```python
from build123d import *

# Parameters (mm, degrees)
SKETCH1_W           = 20
SKETCH1_H           = 6
BOSS_EXTRUDE1_DEPTH = 75
SKETCH2_W           = 20
SKETCH2_H           = 8
BOSS_EXTRUDE2_DEPTH = 26
SKETCH3_W           = 20
SKETCH3_H           = 6
BOSS_EXTRUDE3_DEPTH = 10
SKETCH6_W           = 13
SKETCH6_H           = 13
CUT_EXTRUDE1_DEPTH  = 79.014421744
SKETCH8_R           = 1.5
CUT_EXTRUDE3_DEPTH  = 5
CUT_EXTRUDE4_START  = -5
SKETCH9_R           = 1.5
CUT_EXTRUDE4_DEPTH  = 5
FILLET1_R           = 2
SKETCH10_W          = 6
SKETCH10_H          = 44.050587659
CUT_EXTRUDE5_DEPTH  = 20


with BuildPart() as part:
    # Sketch1 → Boss-Extrude1 (new body)
    with BuildSketch(Plane(origin=(0, 0, 0), x_dir=(1, 0, 0), z_dir=(0, 1, 0))):
        with Locations((-17.5, 0)):
            Rectangle(SKETCH1_W, SKETCH1_H)
    extrude(amount=BOSS_EXTRUDE1_DEPTH)

    # Sketch2 → Boss-Extrude2 (add)
    with BuildSketch(Plane.XY.offset(3)):
        with Locations((-17.5, 71)):
            Rectangle(SKETCH2_W, SKETCH2_H)
    extrude(amount=BOSS_EXTRUDE2_DEPTH)

    # Sketch3 → Boss-Extrude3 (add)
    with BuildSketch(Plane.XZ.offset(-67)):
        with Locations((-17.5, 26)):
            Rectangle(SKETCH3_W, SKETCH3_H)
    extrude(amount=BOSS_EXTRUDE3_DEPTH)

    # Sketch6 → Cut-Extrude1 (cut, through all)
    with BuildSketch(Plane.XZ.offset(-67)):
        with Locations((-17.5, 13)):
            Rectangle(SKETCH6_W, SKETCH6_H)
    extrude(amount=-CUT_EXTRUDE1_DEPTH, mode=Mode.SUBTRACT)

    # Sketch8 → Cut-Extrude3 (cut)
    with BuildSketch(Plane.XY.offset(6.5)):
        with Locations((-17.5, 71)):
            Circle(SKETCH8_R)
    extrude(amount=-CUT_EXTRUDE3_DEPTH, mode=Mode.SUBTRACT)

    # Sketch9 → Cut-Extrude4 (cut)
    with BuildSketch(Plane(origin=(0, 0, 19.5), x_dir=(-1, 0, 0), z_dir=(0, 0, -1)).offset(CUT_EXTRUDE4_START)):
        with Locations(Location((17.5, 71, 0), (0, 0, 180))):
            Circle(SKETCH9_R)
    extrude(amount=CUT_EXTRUDE4_DEPTH, mode=Mode.SUBTRACT)

    # Fillet1
    fillet1_edges = [part.edges().sort_by_distance(p)[0] for p in [
        (-17.5, 67, 3),
        (-17.5, 67, 23),
    ]]
    fillet(fillet1_edges, radius=FILLET1_R)

    # Sketch10 → Cut-Extrude5 (cut)
    with BuildSketch(Plane(origin=(-7.5, 0, 0), x_dir=(0, 0, -1), z_dir=(1, 0, 0))):
        with Locations((0, 21.22470617)):
            Rectangle(SKETCH10_W, SKETCH10_H)
    extrude(amount=-CUT_EXTRUDE5_DEPTH, mode=Mode.SUBTRACT)


solid = part.part
```
Input: part model. Units: mm. Frame: model coordinates. A direction names the side the tool comes from. Round coordinates to 2 decimals unless told otherwise and drop trailing zeros. Order: outer loops, then holes, each group sorted by start corner. A loop starts at its lowest first (then second) coordinate and runs counter-clockwise, first axis right, second up. Notation, with made-up numbers: (34, -9) - (91, -9) arc R29 cw to (91, 20) - close; hole circle Ø2 at (-27.75, 60.5). An arc over 180 degrees is marked (long way). One line per question, with ' | ' between items. Start each with the question number.
1) Cut plane A-A, the plane x = -14.25. Return the cut outline in (y, z).
2) Set-up query: faces 1 (the flat face through (-18, 57, 26)), 2 (the flat face through (-18, 61, 23)), 3 (the flat face through (-18, 71, 1.5)), 4 (the flat face through (-19, 72, 19.5)). Return all of +Z, -Z, +X, -X, +Y, -Y with unobstructed straight access to the full face (end or side cutting, diameter ignored); none if empty.
3) Cut plane C-C, the plane z = 15. Return the cut outline in (x, y).
4) Contact query for flat-ended pins moving along their axis: P1, Ø5, axis at x = -21, z = 27, coming from the -Y side; P2, Ø1, axis at x = -10, z = 10.5, coming from the -Y side. Output: stop coordinate, or through.
5) Cut plane D-D, the plane y = 71. Return the cut outline in (x, z).
6) Cut plane B-B, the plane y = 62.5. Return the cut outline in (x, z), then the cut area to 3 significant figures.
7) Pull-direction query (X, two-part tool) for faces 5 (the flat face through (-18, 66, 29)), 6 (the flat face through (-7.5, 70, 9)), 7 (the cylindrical face through (-18.61, 72.01, 4.04)); classes: +X half, -X half, draft (parallel to the pull), parting line (faces both ways), or undercut.
8) Ray query, probe 1 along X at (y, z) = (71, 4.45); probe 2 along Z at (x, y) = (-20.25, 72); probe 3 along Y at (x, z) = (-17.5, 5.3). Return the intervals inside material, ascending.
Worked out:
1) outline: (43.25, -3) - (75, -3) - (75, 6.5) - (67, 6.5) - (67, 5) arc R2 cw to (65, 3) - (43.25, 3) - close; (57, 23) - (65, 23) arc R2 cw to (67, 21) - (67, 19.5) - (75, 19.5) - (75, 29) - (57, 29) - close
2) face 1: +Z, +X, -X, -Y | face 2: +X, -X, -Y | face 3: none | face 4: +Y, -Y
3) outline: (-27.5, 67) - (-24, 67) - (-24, 75) - (-27.5, 75) - close; (-11, 67) - (-7.5, 67) - (-7.5, 75) - (-11, 75) - close
4) P1: stops at y = 57 | P2: stops at y = 67
5) outline: (-27.5, -3) - (-7.5, -3) - (-7.5, 29) - (-27.5, 29) - close; hole (-24, 6.5) - (-19, 6.5) - (-19, 1.5) - (-16, 1.5) - (-16, 6.5) - (-11, 6.5) - (-11, 19.5) - (-16, 19.5) - (-16, 24.5) - (-19, 24.5) - (-19, 19.5) - (-24, 19.5) - close
6) outline: (-27.5, -3) - (-7.5, -3) - (-7.5, 3) - (-27.5, 3) - close; (-27.5, 23) - (-7.5, 23) - (-7.5, 29) - (-27.5, 29) - close | area: 240 mm^2
7) face 5: draft | face 6: +X half | face 7: undercut
8) probe 1: x = -27.5 to -19, -16 to -7.5 | probe 2: z = -3 to 6.5, 19.5 to 29 | probe 3: y = 67 to 69.5, 72.5 to 75
